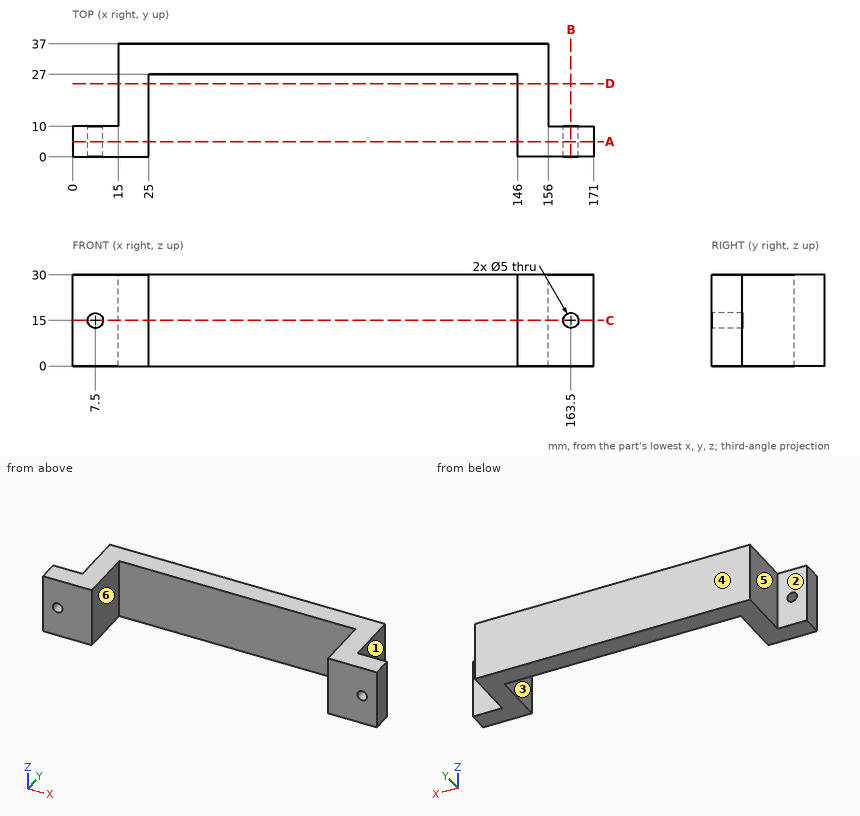
Geometry check sheet. Reference: drawing and pictorial views, mm from the part's lowest x, y, z. A direction names the side the tool comes from. Give positions to 0.01 mm unless a question says otherwise; leave off trailing zeros. Write each loop counter-clockwise with the first axis right and the second up, starting at its lowest first coordinate (ties: lowest second). Pieces come first, ordered by that corner, then holes.
Item 1: Draft check along X on the marked faces 4, 5 and 6. Enter one of: released by +X, released by -X, zero draft, split by the parting line, or undercut.
Item 2: Cross-section at A-A (y = 5). Enter the section's corners in (x, z), and give its area (3 significant figures).
Item 3: Cross-section at C-C (z = 15). Enter the section's corners in (x, y).
Item 4: Cross-section at D-D (y = 24). Enter the section's corners in (x, z).
Item 5: Gauge pin test, flat ends, axial feed: pin 1 (4 mm diameter, centred on y = 16, z = 16, fed in from +X); pin 2 (4.5 mm diameter, centred on x = 9.5, z = 21.5, fed in from +Y); pin 3 (8 mm diameter, centred on x = 140, z = 26.5, fed in from -Y). Record the tip position at first contact, or that the pin passes through.
Item 6: Cross-section at B-B (x = 163.5). Enter the section's corners in (y, z).
Item 7: Scan lines: L1, parallel to X at y = 6.5, z = 15; L2, parallel to X at y = 24.5, z = 6.25; L3, parallel to Z at x = 163.5, y = 5.5. Record each from-to range of solid material in increasing order.
Item 8: Access from +Z, -Z, +X, -X, +Y, -Y to the whole of each face (thin tool, end or side, straight path). Record for the marked faces 1, 2 and 3.
Report:
1. face 4: zero draft
1. face 5: released by -X
1. face 6: undercut
2. outline: (0, 0) - (25, 0) - (25, 30) - (0, 30) - close; (146, 0) - (171, 0) - (171, 30) - (146, 30) - close; hole circle Ø5 at (7.5, 15); hole circle Ø5 at (163.5, 15)
2. area: 1,460 mm2
3. outline: (0, 0) - (5, 0) - (5, 10) - (0, 10) - close; (10, 0) - (25, 0) - (25, 27) - (146, 27) - (146, 0) - (161, 0) - (161, 10) - (156, 10) - (156, 37) - (15, 37) - (15, 10) - (10, 10) - close; (166, 0) - (171, 0) - (171, 10) - (166, 10) - close
4. outline: (15, 0) - (25, 0) - (25, 30) - (15, 30) - close; (146, 0) - (156, 0) - (156, 30) - (146, 30) - close
5. pin 1: stops at x = 156
5. pin 2: stops at y = 10
5. pin 3: stops at y = 27
6. outline: (0, 0) - (10, 0) - (10, 12.5) - (0, 12.5) - close; (0, 17.5) - (10, 17.5) - (10, 30) - (0, 30) - close
7. L1: x = 0 to 5, 10 to 25, 146 to 161, 166 to 171
7. L2: x = 15 to 25, 146 to 156
7. L3: z = 0 to 12.5, 17.5 to 30
8. face 1: +Z, -Z, +X, +Y
8. face 2: +Z, -Z, -X, +Y
8. face 3: +Z, -Z, -Y
